For this review, take the finished solid that the model builds, in its own axes (mm). Coordinates: 2 decimals unless noted, no trailing zeros. Loops run counter-clockwise (first coordinate to the right, second up) from the corner with the lowest first, then second, coordinate; pieces in that order, holes last. Notation, with made-up numbers: (42, 8.5) -> (61, 8.5) arc R21 cw to (61, 19.5) -> close; hole circle Ø5 at (7.5, 24). An arc over 180 degrees is marked (long way). Answer in a Markdown table with one row per item.
from build123d import *

# Parameters (mm, degrees)
SKETCH1_R             = 30
BOSS_EXTRUDE1_DEPTH   = 10
F_8_0MM_DOWEL_HOLE1_D = 8
M6_CLEARANCE_HOLE1_D  = 6.4
CHAMFER1_SIZE         = 0.5


with BuildPart() as part:
    # Sketch1 → Boss-Extrude1 (new body)
    with BuildSketch(Plane(origin=(0, 0, 0), x_dir=(1, 0, 0), z_dir=(0, 1, 0))):
        with Locations(Location((0, 0, 0), (0, 0, 270))):
            Circle(SKETCH1_R)
    extrude(amount=-BOSS_EXTRUDE1_DEPTH)

    # Ø8.0mm Dowel Hole1 (through all)
    with Locations(Plane(origin=(0, 0, 0), x_dir=(1, 0, 0), z_dir=(0, 1, 0))):
        with Locations((-22.5, 0), (22.5, 0)):
            Hole(F_8_0MM_DOWEL_HOLE1_D / 2)

    # M6 Clearance Hole1 (through all)
    with Locations(Plane(origin=(0, 0, 0), x_dir=(1, 0, 0), z_dir=(0, 1, 0))):
        with Locations((19.485571585, -11.25), (-19.485571585, -11.25), (0, 22.5)):
            Hole(M6_CLEARANCE_HOLE1_D / 2)

    # Chamfer1
    chamfer1_edges = [part.edges().sort_by_distance(p)[0] for p in [
        (0, 0, -30),
        (0, -10, -30),
    ]]
    chamfer(chamfer1_edges, length=CHAMFER1_SIZE)


solid = part.part
Item 1: The part is to be moulded in two halves that separate along Z. For faces 1 (the cylindrical face through (25.7, -5.1, 2.4)), 2 (the cylindrical face through (0.417, -5.07, -25.673)), 3 (the flat face through (0, 0, 0)), 4 (the cylindrical face through (1.32, -4.94, -29.97)), say which applies: +Z half, -Z half, draft (parallel to the pull), parting line (faces both ways), or undercut.
Worked answers:
| item | result |
|---|---|
| face 1 | undercut |
| face 2 | undercut |
| face 3 | draft |
| face 4 | parting line |
Item 2: For L1, parallel to X at y = -5.25, z = 11.25; L2, parallel to X at y = -4.5, z = -3; L3, parallel to Z at x = 5.5, y = -9.25, list the stretches that pass through material, from the lowest coordinate up.
Worked answers:
| item | result |
|---|---|
| L1 | -27.81 to -22.69, -16.29 to 16.29, 22.69 to 27.81 |
| L2 | -29.85 to -25.15, -19.85 to 19.85, 25.15 to 29.85 |
| L3 | -29.49 to 29.49 |
Item 3: Take a section at A-A, the plane z = 0. State the section outline as (x, y) points, and give its area (4 significant figures).
Worked answers:
| item | result |
|---|---|
| outline | (-30, -9.5) -> (-29.5, -10) -> (-26.5, -10) -> (-26.5, 0) -> (-29.5, 0) -> (-30, -0.5) -> close; (-18.5, -10) -> (18.5, -10) -> (18.5, 0) -> (-18.5, 0) -> close; (26.5, -10) -> (29.5, -10) -> (30, -9.5) -> (30, -0.5) -> (29.5, 0) -> (26.5, 0) -> close |
| area | 439.5 mm² |
Item 4: Take a section at D-D, the plane z = 12. Count the separate pieces of the cut face and the enclosed holes in it, and give its area (3 significant figures).
Worked answers:
| item | result |
|---|---|
| separate pieces | 3 |
| enclosed holes | 0 |
| area | 425 mm² |
Item 5: Take a section at B-B, the plane x = 0. State the section outline as (y, z) points.
Worked answers:
| item | result |
|---|---|
| outline | (-10, -29.5) -> (-9.5, -30) -> (-0.5, -30) -> (0, -29.5) -> (0, -25.7) -> (-10, -25.7) -> close; (-10, -19.3) -> (0, -19.3) -> (0, 29.5) -> (-0.5, 30) -> (-9.5, 30) -> (-10, 29.5) -> close |
Item 6: Insertion check: pin 1 (9 mm diameter, centred on x = 22.5, z = 0, fed in from +Y); pin 2 (5 mm diameter, centred on x = -22.5, z = 0, fed in from -Y); pin 3 (1 mm diameter, centred on y = -6.5, z = 8.5, fed in from +X); pin 4 (4 mm diameter, centred on y = -4.5, z = -20, fed in from +X). Each pin has a flat end and moves straight along its axis. Give the tip position at first contact, or say it passes through.
Worked answers:
| item | result |
|---|---|
| pin 1 | y = 0 |
| pin 2 | through |
| pin 3 | x = 28.91 |
| pin 4 | x = 24 |
Item 7: Take a section at C-C, the plane y = -2.75. State the section outline as (x, z) points.
Worked answers:
| item | result |
|---|---|
| outline | circle Ø60 at (0, 0); hole circle Ø8 at (-22.5, 0); hole circle Ø6.4 at (-19.49, 11.25); hole circle Ø6.4 at (0, -22.5); hole circle Ø6.4 at (19.49, 11.25); hole circle Ø8 at (22.5, 0) |
